```python
from build123d import *

# Parameters (mm, degrees)
MODEL_W                 = 3
MODEL_H                 = 3
SALIENTE_EXTRUIR1_DEPTH = 1.5


with BuildPart() as part:
    # Model → Saliente-Extruir1 (new body)
    with BuildSketch(Plane.XY):
        with BuildLine():
            Line((12.181222481, 298.136475095), (57.181222481, 298.136475095))
            ThreePointArc((57.181222481, 298.136475095), (61.681222481, 293.636475095), (57.181222481, 289.136475095))
            Line((57.181222481, 289.136475095), (12.181222481, 289.136475095))
            ThreePointArc((12.181222481, 289.136475095), (7.681222481, 293.636475095), (12.181222481, 298.136475095))
        make_face()
        with Locations((12.181222481, 293.636475095)):
            Rectangle(MODEL_W, MODEL_H, mode=Mode.SUBTRACT)
        with Locations((21.181222481, 293.636475095)):
            Rectangle(MODEL_W, MODEL_H, mode=Mode.SUBTRACT)
        with Locations((30.181222481, 293.636475095)):
            Rectangle(MODEL_W, MODEL_H, mode=Mode.SUBTRACT)
        with Locations((39.181222481, 293.636475095)):
            Rectangle(MODEL_W, MODEL_H, mode=Mode.SUBTRACT)
        with Locations((57.181222481, 293.636475095)):
            Rectangle(MODEL_W, MODEL_H, mode=Mode.SUBTRACT)
        with Locations((48.181222481, 293.636475095)):
            Rectangle(MODEL_W, MODEL_H, mode=Mode.SUBTRACT)
    extrude(amount=SALIENTE_EXTRUIR1_DEPTH)


solid = part.part
```
Geometry check sheet. Reference: the model listing, model coordinates, mm. A direction names the side the tool comes from. Round coordinates to 2 decimals unless told otherwise and drop trailing zeros. Loops run counter-clockwise (first coordinate to the right, second up) from the corner with the lowest first, then second, coordinate; pieces in that order, holes last. Notation, with made-up numbers: (17.25, 5.25) - (45.25, 5.25) arc R26 ccw to (45.25, 23.25) - close; hole circle Ø3 at (47.5, -33.75). An arc over 180 degrees is marked (long way). Write item = value, one per line. Start each with the question number.
1. Section check B-B on x = 30. Enter the section's corners in (y, z).
2. Section check D-D on y = 290.75. Enter the section's corners in (x, z), then the cut area to 3 significant figures.
3. Section check C-C on y = 293. Enter the section's corners in (x, z), then the cut area to 3 significant figures.
4. Thickness scan on line 1 (Y direction, x = 30, z = 0.4); line 2 (Y direction, x = 11, z = 0.35); line 3 (X direction, y = 292, z = 0.1). Record the ranges inside material, lowest first.
5. Set-up check for faces 1 (the face through (35, 294, 0)), 2 (the face through (57, 292.136, 1)): record each of +Z, -Z, +X, -X, +Y, -Y from which the full face is reachable in a straight line by a thin tool's end or side.
6. Section check A-A on z = 1.25. Enter the section's corners in (x, y).
Working result:
q1.outline = (289.14, 0) - (292.14, 0) - (292.14, 1.5) - (289.14, 1.5) - close; (295.14, 0) - (298.14, 0) - (298.14, 1.5) - (295.14, 1.5) - close
q2.outline = (8.73, 0) - (60.63, 0) - (60.63, 1.5) - (8.73, 1.5) - close
q2.area = 77.9 mm^2
q3.outline = (7.73, 0) - (10.68, 0) - (10.68, 1.5) - (7.73, 1.5) - close; (13.68, 0) - (19.68, 0) - (19.68, 1.5) - (13.68, 1.5) - close; (22.68, 0) - (28.68, 0) - (28.68, 1.5) - (22.68, 1.5) - close; (31.68, 0) - (37.68, 0) - (37.68, 1.5) - (31.68, 1.5) - close; (40.68, 0) - (46.68, 0) - (46.68, 1.5) - (40.68, 1.5) - close; (49.68, 0) - (55.68, 0) - (55.68, 1.5) - (49.68, 1.5) - close; (58.68, 0) - (61.64, 0) - (61.64, 1.5) - (58.68, 1.5) - close
q3.area = 53.9 mm^2
q4.line_1 = 289.14 to 292.14, 295.14 to 298.14
q4.line_2 = 289.29 to 292.14, 295.14 to 297.98
q4.line_3 = 7.99 to 61.37
q5.face_1 = -Z, +X, -X, +Y, -Y
q5.face_2 = +Z, -Z
q6.outline = (12.18, 289.14) - (57.18, 289.14) arc R4.5 ccw to (57.18, 298.14) - (12.18, 298.14) arc R4.5 ccw to start; hole (10.68, 292.14) - (13.68, 292.14) - (13.68, 295.14) - (10.68, 295.14) - close; hole (19.68, 292.14) - (22.68, 292.14) - (22.68, 295.14) - (19.68, 295.14) - close; hole (28.68, 292.14) - (31.68, 292.14) - (31.68, 295.14) - (28.68, 295.14) - close; hole (37.68, 292.14) - (40.68, 292.14) - (40.68, 295.14) - (37.68, 295.14) - close; hole (46.68, 292.14) - (49.68, 292.14) - (49.68, 295.14) - (46.68, 295.14) - close; hole (55.68, 292.14) - (58.68, 292.14) - (58.68, 295.14) - (55.68, 295.14) - close
